```python
from build123d import *

# Parameters (mm, degrees)
F0_W         = 95.25
F0_H         = 50.8
F1_DEPTH     = 6.35
F2_W         = 82.55
F2_H         = 38.1
F3_DEPTH     = 6.35
F4_R         = 19.05
F5_DEPTH     = 12.7
F5_TAPER     = 10
F6_DEPTH     = 50.8
F6_FACE_R    = 16.810647345
F7_DEPTH     = 12.7
F7_TAPER     = -10
F8_T         = 2.54
F8_T3_DEPTH  = 87.63
F8_T5_DEPTH  = 43.18
F8_T8_ANGLE  = 180.0000001354
F8_T10_ANGLE = 90.000000001
F8_T12_ANGLE = 89.9999998666
F8_T14_ANGLE = 180.000000001
F8_T16_ANGLE = 90.000000001
F8_T18_ANGLE = 90.000000001
F9_R         = 5.08


# Not quite as in the source:
# - a shell that OpenCascade refuses in one call is made with other operations: the cavity is built on its own and cut out


with BuildPart() as f1:
    # F0 (on Top) → F1 (new body)
    with BuildSketch(Plane.XY):
        Rectangle(F0_W, F0_H)
    extrude(amount=F1_DEPTH)

    # F2 (on face) → F3 (join)
    with BuildSketch(Plane.XY.offset(6.35)):
        Rectangle(F2_W, F2_H)
    extrude(amount=F3_DEPTH)

    # F4 (on face) → F5 (join)
    with BuildSketch(Plane.XY.offset(12.7)):
        with Locations((-22.1206657588, 0)):
            Circle(F4_R)
        with Locations((22.1206657588, 0)):
            Circle(F4_R)
    extrude(amount=F5_DEPTH, taper=F5_TAPER)

    # F6 (add): faces of the model
    f6_faces = [f1.faces().sort_by_distance(p)[0] for p in [
        (-22.1206657588, 0, 25.4),
        (22.1206657588, 0, 25.4),
    ]]
    extrude(f6_faces, amount=F6_DEPTH)

    # F6_face (on face) → F7 (join)
    with BuildSketch(Plane(origin=(22.1206657588, 0, 76.2), x_dir=(1, 0, 0), z_dir=(0, 0, 1))):
        Circle(F6_FACE_R)
        with Locations((-44.2413315177, 0)):
            Circle(F6_FACE_R)
    extrude(amount=F7_DEPTH, taper=F7_TAPER)

    # F8: shell of thickness 2.54, made by hand


with BuildPart() as f8_core1:
    # F8_t2: copy of F1
    add(f1.part)

    # the walls: a layer under each face that stays
    f8_faces = [f8_core1.faces().sort_by_distance(p)[0] for p in [
        (0, -25.4, 3.175),
        (-47.625, 0, 3.175),
        (47.625, 0, 3.175),
        (-40.8214285714, -21.7714285714, 6.35),
        (0, 25.4, 3.175),
        (0, -19.05, 9.525),
        (41.275, 0, 9.525),
        (0, 19.05, 9.525),
        (-41.275, 0, 9.525),
        (-38.0826109524, -12.7, 12.7),
        (0, 0, 12.7),
        (38.0826109598, -12.7, 12.7),
        (-40.0509894313, 0, 19.05),
        (4.1903420863, 0, 19.05),
        (-38.9313131039, 0, 50.8),
        (5.3100184138, 0, 50.8),
        (-40.0509894313, 0, 82.55),
        (4.1903420863, 0, 82.55),
    ]]
    thicken(f8_faces, amount=-F8_T, mode=Mode.SUBTRACT)

    # F8_s4 → F8_t3 (cut)
    with BuildSketch(Plane.YZ.offset(-43.815)):
        Polygon((-19.0754, 6.3754), (-19.05, 3.81), (-16.51, 3.81), (-16.51, 6.35), align=None)
        Polygon((19.0754, 6.3754), (19.05, 3.81), (16.51, 3.81), (16.51, 6.35), align=None)
    extrude(amount=F8_T3_DEPTH, mode=Mode.SUBTRACT)

    # F8_s6 → F8_t5 (cut)
    with BuildSketch(Plane.XZ.offset(-21.59)):
        Polygon((41.3004, 6.3754), (41.275, 3.81), (38.735, 3.81), (38.735, 6.35), align=None)
        Polygon((-41.3004, 6.3754), (-41.275, 3.81), (-38.735, 3.81), (-38.735, 6.35), align=None)
    extrude(amount=F8_T5_DEPTH, mode=Mode.SUBTRACT)

    # F8_s7 → F8_t8 (revolve, cut)
    with BuildSketch(Plane.YZ.offset(-22.1206657588)):
        Polygon((-19.0750141169, 12.7298106637), (-19.05, 10.16), (-16.9186869368, 10.16), (-16.5485883073, 12.2589336287), align=None)
    revolve(axis=Axis((-22.1206657588, 0, 12.7), (0, 0, -1)), revolution_arc=F8_T8_ANGLE, mode=Mode.SUBTRACT)

    # F8_s9 → F8_t10 (revolve, cut)
    with BuildSketch(Plane.XZ):
        Polygon((-3.0456516419, 12.7298106637), (-3.0706657588, 10.16), (-5.201978822, 10.16), (-5.5720774515, 12.2589336287), align=None)
    revolve(axis=Axis((-22.1206657588, 0, 12.7), (0, 0, -1)), revolution_arc=F8_T10_ANGLE, mode=Mode.SUBTRACT)

    # F8_s11 → F8_t12 (revolve, cut)
    with BuildSketch(Plane.YZ.offset(-22.1206657588)):
        Polygon((19.0750141169, 12.7298106637), (19.05, 10.16), (16.9186869368, 10.16), (16.5485883073, 12.2589336287), align=None)
    revolve(axis=Axis((-22.1206657588, 0, 12.7), (0, 0, -1)), revolution_arc=F8_T12_ANGLE, mode=Mode.SUBTRACT)

    # F8_s13 → F8_t14 (revolve, cut)
    with BuildSketch(Plane.YZ.offset(22.1206657588)):
        Polygon((-19.0750141169, 12.7298106637), (-19.05, 10.16), (-16.9186869368, 10.16), (-16.5485883073, 12.2589336287), align=None)
    revolve(axis=Axis((22.1206657588, 0, 12.7), (0, 0, -1)), revolution_arc=F8_T14_ANGLE, mode=Mode.SUBTRACT)

    # F8_s15 → F8_t16 (revolve, cut)
    with BuildSketch(Plane.XZ):
        Polygon((41.1956798758, 12.7298106637), (41.1706657588, 10.16), (39.0393526957, 10.16), (38.6692540662, 12.2589336287), align=None)
    revolve(axis=Axis((22.1206657588, 0, 12.7), (0, 0, -1)), revolution_arc=F8_T16_ANGLE, mode=Mode.SUBTRACT)

    # F8_s17 → F8_t18 (revolve, cut)
    with BuildSketch(Plane.YZ.offset(22.1206657588)):
        Polygon((19.0750141169, 12.7298106637), (19.05, 10.16), (16.9186869368, 10.16), (16.5485883073, 12.2589336287), align=None)
    revolve(axis=Axis((22.1206657588, 0, 12.7), (0, 0, -1)), revolution_arc=F8_T18_ANGLE, mode=Mode.SUBTRACT)

    # F8_s19 → F8_t20 (revolve, cut)
    with BuildSketch(Plane.XZ):
        Polygon((-5.2596042969, 25.4044106637), (-7.8114301065, 24.9589336287), (-7.8500184138, 25.1777787946), (-7.8500184138, 25.4), align=None)
    revolve(axis=Axis((-22.1206657588, 0, 25.4), (0, 0, -1)), mode=Mode.SUBTRACT)

    # F8_s21 → F8_t22 (revolve, cut)
    with BuildSketch(Plane.XZ):
        Polygon((38.9817272208, 25.4044106637), (36.4299014112, 24.9589336287), (36.3913131039, 25.1777787946), (36.3913131039, 25.4), align=None)
    revolve(axis=Axis((22.1206657588, 0, 25.4), (0, 0, -1)), mode=Mode.SUBTRACT)

    # F8_s23 → F8_t24 (revolve, cut)
    with BuildSketch(Plane.XZ):
        Polygon((-5.2596042969, 76.1955893363), (-7.8500184138, 76.2), (-7.8500184138, 76.4222212054), (-7.8114301065, 76.6410663713), align=None)
    revolve(axis=Axis((-22.1206657588, 0, 76.2), (0, 0, -1)), mode=Mode.SUBTRACT)

    # F8_s25 → F8_t26 (revolve, cut)
    with BuildSketch(Plane.XZ):
        Polygon((38.9817272208, 76.1955893363), (36.3913131039, 76.2), (36.3913131039, 76.4222212054), (36.4299014112, 76.6410663713), align=None)
    revolve(axis=Axis((22.1206657588, 0, 76.2), (0, 0, -1)), mode=Mode.SUBTRACT)


with BuildPart() as f1_1:
    add(f1.part)

    # what is left inside the walls is the cavity
    f8_cavity = [f8_core1.part.solids().sort_by_distance(p)[0] for p in [
        (-36.365913, 0, 59.266667),
    ]]
    add(f8_cavity, mode=Mode.SUBTRACT)

    # F9
    f9_edges = [f1_1.edges().sort_by_distance(p)[0] for p in [
        (-47.625, -25.4, 3.175),
        (47.625, -25.4, 3.175),
        (47.625, 25.4, 3.175),
        (-47.625, 25.4, 3.175),
    ]]
    fillet(f9_edges, radius=F9_R)


solid = f1_1.part
```
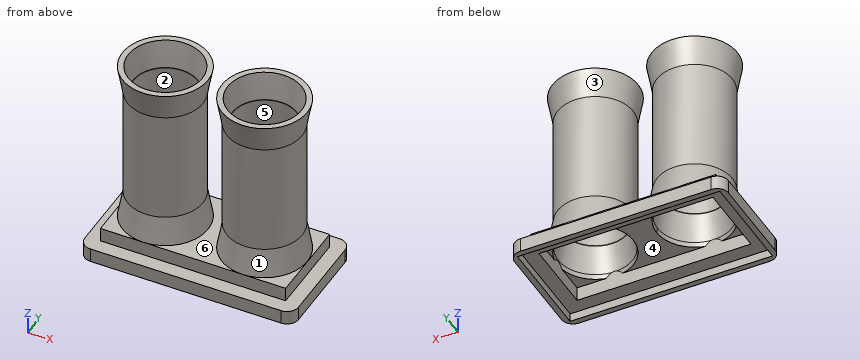
Check sheet for the modelled part. Datum: model origin and axes. Units: mm. Face numbers are marked on the shaded views. A direction names the side the tool comes from. Give positions to 0.01 mm unless a question says otherwise; leave off trailing zeros. Write each loop counter-clockwise with the first axis right and the second up, starting at its lowest first coordinate (ties: lowest second). Pieces come first, ordered by that corner, then holes. Notation, with made-up numbers: (50, 20.5) - (55, 20.5) arc R7 cw to (55, 26.5) - close; hole circle Ø1 at (57, 30.25). An arc over 180 degrees is marked (long way). Answer as a JSON object with one key per item and string values. Group by question number.
1) Sectioned sample at B-B (x = 1.5). Record the cut outline in (y, z).
2) Sectioned sample at C-C (y = 5). Give the number of separate pieces and of enclosed holes in the cut face, then the cut area to 3 significant figures.
3) Access from +Z, -Z, +X, -X, +Y, -Y to the whole of each face (thin tool, end or side, straight path). Record for the marked faces 1 and 2.
4) Depth check by flat-ended pin: P1, Ø2, axis at x = 0.5, y = 17.5, coming from the -Z side; P2, Ø1, axis at x = 12.5, z = 48.5, coming from the +Y side; P3, Ø2, axis at y = 2, z = 73.5, coming from the +X side; P4, Ø4, axis at x = -30, y = 8, coming from the -Z side. Enter the tip coordinate at first touch or a pass-through.
5) Release check for a two-part mould opening along Y. For the marked faces 3, 4, 5 and 6 record: pulls with the +Y half, pulls with the -Y half, needs draft (parallel to the pull), parting line crosses it, or undercut.
6) Thickness scan on probe 1 along X at (y, z) = (0, 45); probe 2 along Y at (x, z) = (-21, 10.5); probe 3 along X at (y, z) = (-2, 29). Record the ranges inside material, lowest first. Write a range as from..to.
7) Sectioned sample at A-A (z = 62.5). Record the cut outline in (x, y).
Geometry results:
{
 "1": {"outline": "(-25.4, 0) - (-22.86, 0) - (-22.86, 3.81) - (-16.51, 3.81) - (-16.51, 10.16) - (16.51, 10.16) - (16.51, 3.81) - (22.86, 3.81) - (22.86, 0) - (25.4, 0) - (25.4, 6.35) - (19.05, 6.35) - (19.05, 12.7) - (-19.05, 12.7) - (-19.05, 6.35) - (-25.4, 6.35) - close"},
 "2": {"separate pieces": "3", "enclosed holes": "0", "area": "952 mm^2"},
 "3": {"face 1": "none", "face 2": "+Z, -Z"},
 "4": {"P1": "stops at z = 3.81", "P2": "stops at y = 14.12", "P3": "stops at x = 38.9", "P4": "passes through"},
 "5": {"face 3": "parting line crosses it", "face 4": "undercut", "face 5": "undercut", "face 6": "needs draft"},
 "6": {"probe 1": "x = -38.93..-36.39, -7.85..-5.31, 5.31..7.85, 36.39..38.93", "probe 2": "y = -19.05..-16.51, 16.51..19.05", "probe 3": "x = -38.81..-36.25, -7.99..-5.43, 5.43..7.99, 36.25..38.81"},
 "7": {"outline": "circle Ø33.62 at (-22.12, 0); circle Ø33.62 at (22.12, 0); hole circle Ø28.54 at (-22.12, 0); hole circle Ø28.54 at (22.12, 0)"}
}
